```python
from build123d import *

# Parameters (mm, degrees)
BOSS_EXTRUDE2_DEPTH = 25.4
SKETCH2_W           = 64.689945596
SKETCH2_H           = 22.4536
CUT_EXTRUDE1_DEPTH  = 51.521177338
SKETCH5_R           = 3.302
CUT_EXTRUDE2_DEPTH  = 43.38328072


with BuildPart() as part:
    # Sketch1 → Boss-Extrude2 (new body)
    with BuildSketch(Plane(origin=(0, 0, 0), x_dir=(1, 0, 0), z_dir=(0, 1, 0))):
        with BuildLine():
            Line((15.875, 14.111111111), (15.875, 0))
            Line((15.875, 0), (0, 0))
            Line((0, 0), (-15.875, 0))
            Line((-15.875, 0), (-15.875, 14.111111111))
            ThreePointArc((-15.875, 14.111111111), (0, 29.986111111), (15.875, 14.111111111))
        make_face()
    extrude(amount=BOSS_EXTRUDE2_DEPTH)

    # Sketch2 → Cut-Extrude1 (cut, through all)
    with BuildSketch(Plane(origin=(15.875, 0, 0), x_dir=(0, 0, -1), z_dir=(1, 0, 0))):
        with Locations((33.818172798, 12.7)):
            Rectangle(SKETCH2_W, SKETCH2_H)
    extrude(amount=-CUT_EXTRUDE1_DEPTH, mode=Mode.SUBTRACT)

    # Sketch5 → Cut-Extrude2 (cut, through all)
    with BuildSketch(Plane.XZ):
        with Locations(Location((0, -17.78, 0), (0, 0, 270))):
            Circle(SKETCH5_R)
    extrude(amount=-CUT_EXTRUDE2_DEPTH, mode=Mode.SUBTRACT)


solid = part.part
```
For this review, take the finished solid that the model builds, in its own axes (mm). A direction names the side the tool comes from. Round coordinates to 2 decimals unless told otherwise and drop trailing zeros. Write each loop counter-clockwise with the first axis right and the second up, starting at its lowest first coordinate (ties: lowest second). Pieces come first, ordered by that corner, then holes. Notation, with made-up numbers: (49, 72.25) - (104, 72.25) arc R27 ccw to (104, 91.25) - close; hole circle Ø10 at (24, -27.5). An arc over 180 degrees is marked (long way). Put each result on its own line as item: value.
Q1. We need section C-C (z = -17.78). Give the boundary of the cut face in (x, y).
Solved:
outline: (-15.45, 0) - (-3.3, 0) - (-3.3, 1.47) - (-15.45, 1.47) - close; (-15.45, 23.93) - (-3.3, 23.93) - (-3.3, 25.4) - (-15.45, 25.4) - close; (3.3, 0) - (15.45, 0) - (15.45, 1.47) - (3.3, 1.47) - close; (3.3, 23.93) - (15.45, 23.93) - (15.45, 25.4) - (3.3, 25.4) - close
Q2. Insertion check: pin 1 Ø8 at (x, y) = (12.5, 13.5) entering from -Z; pin 2 Ø4 at (x, z) = (0, -17.78) entering from +Y. Each pin has a flat end and moves straight along its axis. Give the tip position at first contact, or say it passes through.
Solved:
pin 1: stops at z = -1.47
pin 2: passes through
Q3. We need section A-A (x = 0). Give the boundary of the cut face in (y, z).
Solved:
outline: (0, -29.99) - (1.47, -29.99) - (1.47, -21.08) - (0, -21.08) - close; (0, -14.48) - (1.47, -14.48) - (1.47, -1.47) - (23.93, -1.47) - (23.93, -14.48) - (25.4, -14.48) - (25.4, 0) - (0, 0) - close; (23.93, -29.99) - (25.4, -29.99) - (25.4, -21.08) - (23.93, -21.08) - close
Q4. Mouldability with a two-part tool opening along Y and no side actions: class faces 3 (the face through (0, 13, 0)), 4 (the face through (0, 13, -1.473)), 5 (the face through (0, 1.473, -12)), 6 (the face through (0, 25.4, -12)) as released by +Y, released by -Y, zero draft, split by the parting line, or undercut.
Solved:
face 3: zero draft
face 4: undercut
face 5: undercut
face 6: released by +Y
Q5. We need section D-D (x = 6). Give the boundary of the cut face in (y, z), and give its area (3 significant figures).
Solved:
outline: (0, -28.81) - (1.47, -28.81) - (1.47, -1.47) - (23.93, -1.47) - (23.93, -28.81) - (25.4, -28.81) - (25.4, 0) - (0, 0) - close
area: 118 mm2
Q6. Wall thickness on probe 1 along Y at (x, z) = (10.5, -12.75); probe 2 along Z at (x, y) = (8, 13.75); probe 3 along X at (y, z) = (24.45, -17.78): over which ranges is each line inside the solid? List them lowest first.
Solved:
probe 1: y = 0 to 1.47, 23.93 to 25.4
probe 2: z = -1.47 to 0
probe 3: x = -15.45 to -3.3, 3.3 to 15.45
Q7. We need section B-B (z = -2.75). Give the boundary of the cut face in (x, y) (3 decimals).
Solved:
outline: (-15.875, 0) - (15.875, 0) - (15.875, 1.473) - (-15.875, 1.473) - close; (-15.875, 23.927) - (15.875, 23.927) - (15.875, 25.4) - (-15.875, 25.4) - close
Q8. Machinability: for faces 1 (the face through (0, 23.927, -12)), 2 (the face through (-0.349, 0.726, -29.982)), which of the approach directions +Z, -Z, +X, -X, +Y, -Y give a long, thin tool a straight path to every point of the face, cutting with its end or side? Answer none if there is none.
Solved:
face 1: -Z, +X, -X
face 2: -Z, +Y, -Y
